The figure shows three views and two pictorial views of one solid part (mm, origin at its lowest corner). Answer the questions. A direction names the side the tool comes from. Round coordinates to 2 decimals unless told otherwise and drop trailing zeros. Order: outer loops, then holes, each group sorted by start corner. A loop starts at its lowest first (then second) coordinate and runs counter-clockwise, first axis right, second up. Notation, with made-up numbers: (47, 69.25) - (73, 69.25) arc R28 ccw to (73, 96.25) - close; hole circle Ø9 at (37.5, -30.75). An arc over 180 degrees is marked (long way). Answer in a Markdown table with one row per item.
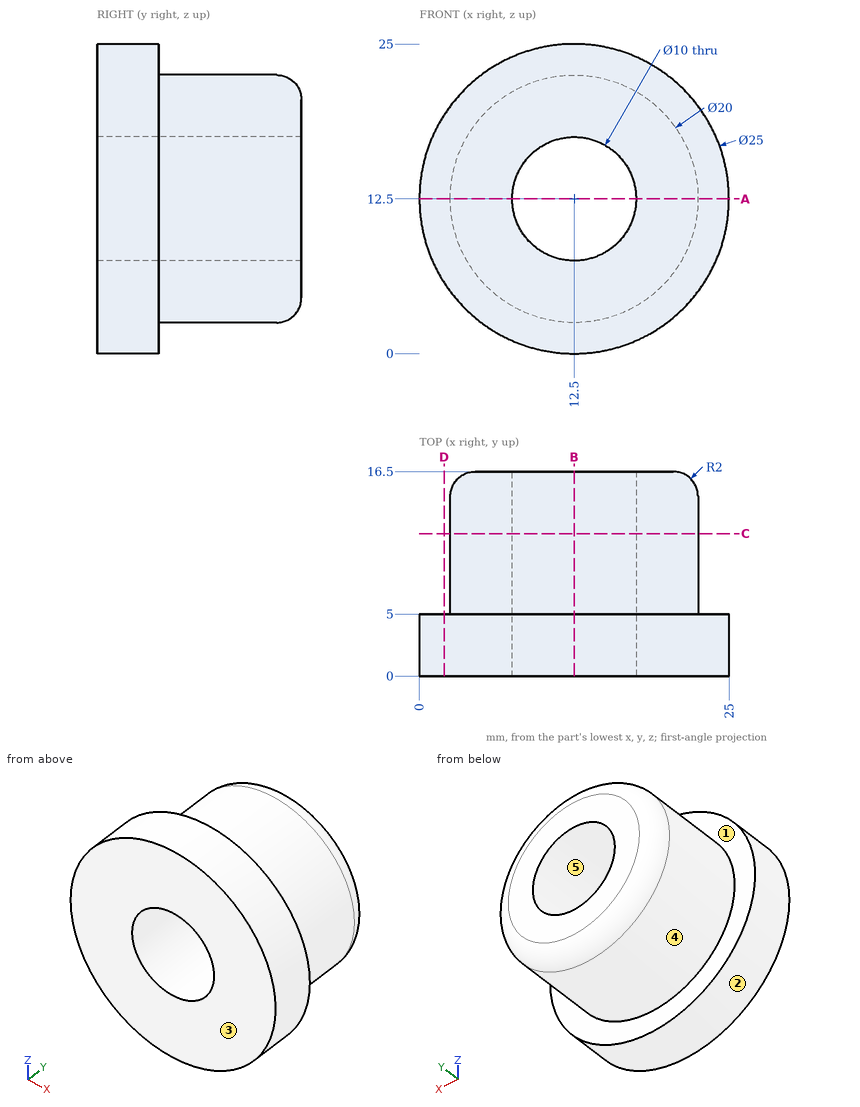
1) Find section B-B, the plane x = 12.5. Give the vertices of the cut face in (y, z), then the cut area to 3 significant figures.
Filled in:
| item | result |
|---|---|
| outline | (0, 0) - (5, 0) - (5, 2.5) - (14.5, 2.5) arc R2 ccw to (16.5, 4.5) - (16.5, 7.5) - (0, 7.5) - close; (0, 17.5) - (16.5, 17.5) - (16.5, 20.5) arc R2 ccw to (14.5, 22.5) - (5, 22.5) - (5, 25) - (0, 25) - close |
| area | 188 mm^2 |
2) The mould has two halves that part along Z. Classify the marked faces 3, 4 and 5: released by +Z, released by -Z, zero draft, split by the parting line, or undercut.
Filled in:
| item | result |
|---|---|
| face 3 | zero draft |
| face 4 | split by the parting line |
| face 5 | undercut |
3) Find the intervals of material crossed by probe 1 along Z at (x, y) = (12.5, 6.25); probe 2 along Z at (x, y) = (12.5, 3.5); probe 3 along Y at (x, z) = (9.25, 2), in increasing order. Write a range as from..to.
Filled in:
| item | result |
|---|---|
| probe 1 | z = 2.5..7.5, 17.5..22.5 |
| probe 2 | z = 0..7.5, 17.5..25 |
| probe 3 | y = 0..5 |
4) Find section C-C, the plane y = 11.5. Give the vertices of the cut face in (x, z).
Filled in:
| item | result |
|---|---|
| outline | circle Ø20 at (12.5, 12.5); hole circle Ø10 at (12.5, 12.5) |
5) Which of the six approach directions +Z, -Z, +X, -X, +Y, -Y give full straight-line access (tool end or side, diameter ignored) to the marked faces 1 and 2?
Filled in:
| item | result |
|---|---|
| face 1 | +Y |
| face 2 | +Y, -Y |
6) Find section D-D, the plane x = 2. Give the vertices of the cut face in (y, z), then the cut area to 3 significant figures.
Filled in:
| item | result |
|---|---|
| outline | (0, 5.72) - (5, 5.72) - (5, 19.28) - (0, 19.28) - close |
| area | 67.8 mm^2 |
7) Each of these flat-tipped pins is pushed along its axis until it touches: pin 1 (1.5 mm diameter, centred on y = 10, z = 11.5, fed in from -X); pin 2 (1 mm diameter, centred on x = 9.5, z = 5.5, fed in from -Y); pin 3 (2 mm diameter, centred on x = 4.5, z = 19.5, fed in from +Y); pin 4 (1.5 mm diameter, centred on y = 3, z = 16.5, fed in from +X). Where does it stop, or does it pass through?
Filled in:
| item | result |
|---|---|
| pin 1 | stops at x = 2.5 |
| pin 2 | stops at y = 0 |
| pin 3 | stops at y = 15.66 |
| pin 4 | stops at x = 24.57 |
8) Find section A-A, the plane z = 12.5. Give the vertices of the cut face in (x, y), then the cut area to 3 significant figures.
Filled in:
| item | result |
|---|---|
| outline | (0, 0) - (7.5, 0) - (7.5, 16.5) - (4.5, 16.5) arc R2 ccw to (2.5, 14.5) - (2.5, 5) - (0, 5) - close; (17.5, 0) - (25, 0) - (25, 5) - (22.5, 5) - (22.5, 14.5) arc R2 ccw to (20.5, 16.5) - (17.5, 16.5) - close |
| area | 188 mm^2 |
